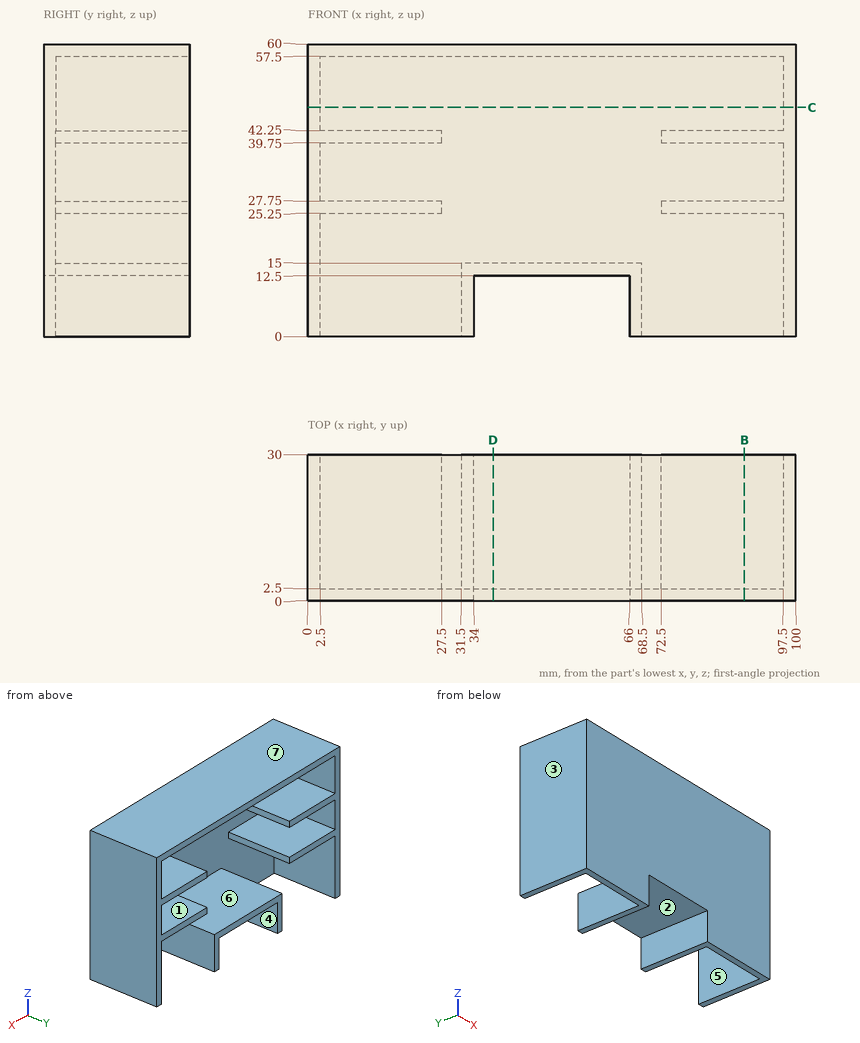
Could you check a few things on this drawing? It's one solid part, dimensions in mm from its lowest x, y, z. A direction names the side the tool comes from. Coordinates: 2 decimals unless noted, no trailing zeros. Order: outer loops, then holes, each group sorted by start corner. A loop starts at its lowest first (then second) coordinate and runs counter-clockwise, first axis right, second up. Notation, with made-up numbers: (70.25, -3) -> (100.25, -3) arc R26 cw to (100.25, 14) -> close; hole circle Ø11 at (62, 63). An arc over 180 degrees is marked (long way). Answer in a Markdown table with one row per item.
(1) I want a section at D-D on x = 38. List the corners of the cut face in (y, z) for me, then the cut area to 3 significant figures.
Answer key:
| item | result |
|---|---|
| outline | (0, 12.5) -> (30, 12.5) -> (30, 15) -> (2.5, 15) -> (2.5, 57.5) -> (30, 57.5) -> (30, 60) -> (0, 60) -> close |
| area | 256 mm^2 |
(2) Thinking about a two-plate mould opening in Z: for the marked faces 1, 2 and 3, which applies, +Z half, -Z half, draft (parallel to the pull), parting line (faces both ways), or undercut?
Answer key:
| item | result |
|---|---|
| face 1 | undercut |
| face 2 | -Z half |
| face 3 | draft |
(3) I want a section at C-C on z = 47. List the corners of the cut face in (x, y) for me.
Answer key:
| item | result |
|---|---|
| outline | (0, 0) -> (100, 0) -> (100, 30) -> (97.5, 30) -> (97.5, 2.5) -> (2.5, 2.5) -> (2.5, 30) -> (0, 30) -> close |
(4) I want a section at B-B on x = 89.5. List the corners of the cut face in (y, z) for me, then the cut area to 3 significant figures.
Answer key:
| item | result |
|---|---|
| outline | (0, 0) -> (2.5, 0) -> (2.5, 25.25) -> (30, 25.25) -> (30, 27.75) -> (2.5, 27.75) -> (2.5, 39.75) -> (30, 39.75) -> (30, 42.25) -> (2.5, 42.25) -> (2.5, 57.5) -> (30, 57.5) -> (30, 60) -> (0, 60) -> close |
| area | 356 mm^2 |
(5) Please list where these lines run through material, in increasing order: probe 1 along X at (y, z) = (28.5, 7.5); probe 2 along Z at (x, y) = (22, 4.5); probe 3 along X at (y, z) = (20.75, 35.5).
Answer key:
| item | result |
|---|---|
| probe 1 | 0 to 2.5, 31.5 to 34, 66 to 68.5, 97.5 to 100 |
| probe 2 | 25.25 to 27.75, 39.75 to 42.25, 57.5 to 60 |
| probe 3 | 0 to 2.5, 97.5 to 100 |
(6) On a 3-axis mill with a long thin cutter (end or side, diameter ignored), from which of +Z, -Z, +X, -X, +Y, -Y can I reach the whole of each face in a straight line? I mean the marked faces 4, 5, 6 and 7. Say none if no direction works.
Answer key:
| item | result |
|---|---|
| face 4 | -Z, +Y, -Y |
| face 5 | -Z, +Y |
| face 6 | +Y |
| face 7 | +Z, +X, -X, +Y, -Y |
(7) Will this pin go through, and if not, where does the flat tip stop? pin 1 Ø1.2 at (y, z) = (16.5, 41) entering from -X.
Answer key:
| item | result |
|---|---|
| pin 1 | x = 0 |
